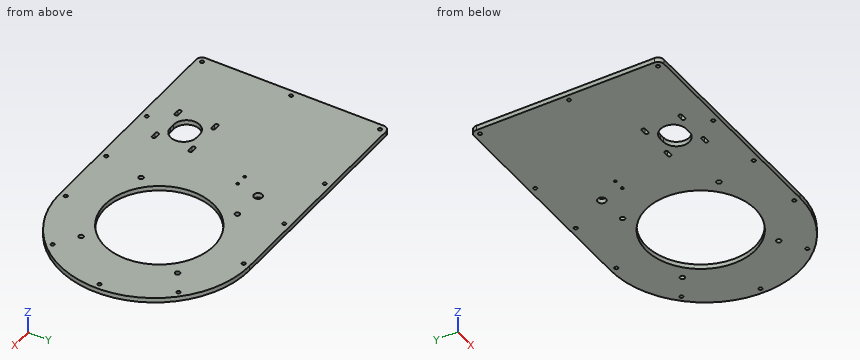
Autodesk Inventor part; units mm, degrees
ref_plane "YZ Plane" through (0, 0, 0) normal (1, 0, 0) x (0, 1, 0)
ref_plane "XZ Plane" through (0, 0, 0) normal (0, 1, 0) x (-1, 0, 0)
ref_plane "XY Plane" through (0, 0, 0) normal (0, 0, 1) x (1, 0, 0)
sketch "Sketch1" plane through (0, 0, 0) normal (0, 0, 1) x (1, 0, 0)
  line L0 (-150, -80) -> (40, -80)
  line L1 (40, 80) -> (-150, 80)
  line L2 (-150, 80) -> (-150, -80)
  line L3 (-150, 0) -> (-107, 0) construction
  line L4 (-107, 0) -> (33.79, 0) construction
  line L5 (33.79, -40.6) -> (33.79, 40.6) construction
  line L6 (-6.81, 0) -> (74.39, 0) construction
  line L7 (33.79, 40.6) -> (74.39, 40.6) construction
  line L8 (74.39, 40.6) -> (74.39, 0) construction
  circle A0 centre (74.39, 40.6) radius 2
  circle A1 centre (74.39, -40.6) radius 2
  circle A2 centre (-6.81, 40.6) radius 2
  circle A3 centre (-6.81, -40.6) radius 2
  line L9 (33.79, 0) -> (33.79, 47) construction
  line L10 (33.79, 0) -> (33.79, -47) construction
  line L11 (-107, -80) -> (-107, -42.5) construction
  line L12 (-107, -42.5) -> (-71.7142, -42.5) construction
  line L13 (33.79, 0) -> (-69.7142, -42.5) construction
  circle A4 centre (-69.7142, -42.5) radius 11 construction
  line L14 (150, 0) -> (120, 0) construction
  line L15 (120, 0) -> (120, 0)
  arc A5 (40, -80) -> (120, 0) centre (40, 0) ccw
  arc A6 (120, 0) -> (40, 80) centre (40, 0) ccw
  line L16 (120, 0) -> (115, 0) construction
  circle A7 centre (115, 0) radius 1.5
  line L17 (40, 0) -> (96.5685, 56.5685) construction
  line L18 (96.5685, -56.5685) -> (93.033, -53.033) construction
  circle A8 centre (93.033, -53.033) radius 1.5
  line L19 (40, -80) -> (40, -75) construction
  circle A9 centre (40, -75) radius 1.5
  line L20 (40, -75) -> (-15, -75) construction
  line L21 (-15, -75) -> (-70, -75) construction
  line L22 (-150, -75) -> (-145, -75) construction
  circle A10 centre (-15, -75) radius 1.5
  circle A11 centre (-70, -75) radius 1.5
  circle A12 centre (-145, -75) radius 1.5
  circle A13 centre (-145, 0) radius 1.5
  circle A14 centre (93.033, 53.033) radius 1.5
  circle A15 centre (40, 75) radius 1.5
  circle A16 centre (-15, 75) radius 1.5
  circle A17 centre (-70, 75) radius 1.5
  circle A18 centre (-145, 75) radius 1.5
  line L23 (-145, -80) -> (-145, -75) construction
  line L24 (-150, 0) -> (-145, 0) construction
  line L25 (-71.7142, -42.5) -> (-67.7142, -42.5) construction
  line L26 (-85.2142, -42.5) -> (-54.2142, -42.5) construction
  line L27 (-69.7142, -27) -> (-69.7142, -58) construction
  line L28 (-69.7142, -27) -> (-85.2142, -27) construction
  line L29 (-85.2142, -27) -> (-85.2142, -42.5) construction
  circle A19 centre (-85.2142, -27) radius 1.5 construction
  circle A20 centre (-54.2142, -27) radius 1.5 construction
  circle A21 centre (-54.2142, -58) radius 1.5 construction
  circle A22 centre (-85.2142, -58) radius 1.5 construction
  line L30 (33.79, 0) -> (31.29, 0) construction
  line L31 (33.79, 0) -> (45.79, 0) construction
  line L32 (45.79, 0) -> (45.79, 58) construction
  circle A23 centre (45.79, 58) radius 1.1
  circle A24 centre (45.79, 65) radius 1.1
  line L33 (-83.2142, -27) -> (-87.2142, -27) construction
  arc A25 (-83.2142, -28.5) -> (-83.2142, -25.5) centre (-83.2142, -27) ccw
  line L34 (-83.2142, -28.5) -> (-87.2142, -28.5)
  line L35 (-83.2142, -25.5) -> (-87.2142, -25.5)
  arc A26 (-87.2142, -25.5) -> (-87.2142, -28.5) centre (-87.2142, -27) ccw
  circle A27 centre (-54.2142, -27) radius 1.5 construction
  line L36 (-56.2142, -27) -> (-52.2142, -27) construction
  arc A28 (-56.2142, -25.5) -> (-56.2142, -28.5) centre (-56.2142, -27) ccw
  line L37 (-56.2142, -28.5) -> (-52.2142, -28.5)
  line L38 (-56.2142, -25.5) -> (-52.2142, -25.5)
  arc A29 (-52.2142, -28.5) -> (-52.2142, -25.5) centre (-52.2142, -27) ccw
  line L39 (-69.7142, -58) -> (-85.2142, -58) construction
  circle A30 centre (-85.2142, -58) radius 1.5 construction
  circle A31 centre (-54.2142, -58) radius 1.5 construction
  line L40 (-83.2142, -58) -> (-87.2142, -58) construction
  arc A32 (-83.2142, -59.5) -> (-83.2142, -56.5) centre (-83.2142, -58) ccw
  line L41 (-83.2142, -56.5) -> (-87.2142, -56.5)
  line L42 (-83.2142, -59.5) -> (-87.2142, -59.5)
  arc A33 (-87.2142, -56.5) -> (-87.2142, -59.5) centre (-87.2142, -58) ccw
  line L43 (-56.2142, -56.5) -> (-52.2142, -56.5)
  arc A34 (-52.2142, -59.5) -> (-52.2142, -56.5) centre (-52.2142, -58) ccw
  line L44 (-56.2142, -58) -> (-52.2142, -58) construction
  circle A35 centre (-54.2142, -58) radius 1.5 construction
  line L45 (-56.2142, -59.5) -> (-52.2142, -59.5)
  arc A36 (-56.2142, -56.5) -> (-56.2142, -59.5) centre (-56.2142, -58) ccw
  arc A37 (-71.7142, -31.5) -> (-71.7142, -53.5) centre (-71.7142, -42.5) ccw
  arc A38 (-67.7142, -53.5) -> (-67.7142, -31.5) centre (-67.7142, -42.5) ccw
  line L46 (-67.7142, -31.5) -> (-71.7142, -31.5)
  line L47 (-67.7142, -53.5) -> (-71.7142, -53.5)
  circle A39 centre (-37.21, 22) radius 1.1
  circle A40 centre (-46.71, 22) radius 1.1
  circle A41 centre (-32.71, 42) radius 3.5
  circle A42 centre (33.79, 0) radius 46
  point P0 (0, 0)
  point P1 (120, -80)
  point P2 (120, 0)
  dimension "d4" = 43
  dimension "d6" = 140.79
  dimension "L_furos" = 81.2
  dimension "d9" = 81.2
  dimension "d11" = 4
  dimension "d30" = 47
  dimension "d40" = 37.5
  dimension "d45" = 111.89
  dimension "DN" = 22
  dimension "d47" = 30
  dimension "d49" = 80
  dimension "LF" = 5
  dimension "Furos" = 3
  dimension "d52" = 45
  dimension "d53" = 5
  dimension "d55" = 3
  dimension "d56" = 5
  dimension "d57" = 3
  dimension "d58" = 55
  dimension "d59" = 55
  dimension "d60" = 5
  dimension "d61" = 3
  dimension "d62" = 3
  dimension "d63" = 3
  dimension "d64" = 3
  dimension "d65" = 5
  dimension "d66" = 5
  dimension "d67" = 33.79
  dimension "d68" = 4
  dimension "d69" = 31
  dimension "d70" = 31
  dimension "FN" = 3
  dimension "d72" = 2.5
  dimension "d77" = 12
  dimension "NN" = 4
  dimension "d84" = 3
  dimension "d85" = 1.5
  dimension "d86" = 22
  dimension "d88" = 11
  dimension "d89" = 43
  dimension "d90" = 58
  dimension "d91" = 7
  dimension "d92" = 2.2
  dimension "d93" = 2.2
  dimension "d94" = 80
  dimension "d95" = 80
  dimension "d96" = 40
  dimension "d97" = 150
  dimension "d98" = 2.2
  dimension "d99" = 2.2
  dimension "d100" = 9.5
  dimension "d101" = 22
  dimension "d102" = 71
  dimension "d103" = 20
  dimension "d104" = 7
  dimension "d106" = 14
  dimension "d107" = 92
extrude "Extrusion1" add sketch "Sketch1" along normal blind 4 contours L2 L1 A6 A5 L0 | A23 | A24 | A39 | A40 | A41
extrude "Extrusion5" cut sketch "Sketch1" along normal up to surface (4 mm away) contours A39 | A40 | A41
fillet "Fillet1" radius 5 2 edges at (-150, -80, 2) (-150, 80, 2)
equation "\"d9\" = L_furos"
equation "\"d53\" = LF"
equation "\"d55\" = Furos"
equation "\"d56\" = LF"
equation "\"d57\" = Furos"
equation "\"d60\" = LF"
equation "\"d61\" = Furos"
equation "\"d62\" = Furos"
equation "\"d63\" = Furos"
equation "\"d64\" = Furos"
equation "\"d65\" = LF"
equation "\"d66\" = LF"
properties part number "Base_solida_TestBR" material "Acrilico"
Model file for the job. Use its own axes, mm. Coordinates: 2 decimals unless noted, no trailing zeros. Loops run counter-clockwise (first coordinate to the right, second up) from the corner with the lowest first, then second, coordinate; pieces in that order, holes last. Notation, with made-up numbers: (0.5, 55.25) - (40.5, 55.25) arc R7 ccw to (40.5, 68.25) - close; hole circle Ø4 at (33.5, -28). An arc over 180 degrees is marked (long way). Answer as a JSON object with one key per item and string values. Group by question number.
(1) Cut at C-C (z = 3.2). State how many separate pieces and enclosed holes the cut face has, then the cut area to 3 significant figures.
(2) Cut at A-A (x = 33.79). Give the cut face in (y, z), then the cut area to 3 significant figures.
(3) Cut at B-B (y = 12). Give the cut face in (x, z).
(4) Cut at D-D (y = 61). Give the cut face in (x, z).
(5) Probe line 1 along Y through (x, z) = (-70, 1.8); line 2 along Y through (x, z) = (74.39, 2.85); line 3 along Y through (x, z) = (-37.21, 1.3). List the from-to ranges inside material, lowest first.
(6) Flat gauge pin, fed straight in: pin 1 (12 mm diameter, centred on x = 17, y = 32, fed in from -Z) (3 decimals). Where does the tip first touch, or does it go through?
Geometry says:
{
 "1": {"separate pieces": "1", "enclosed holes": "25", "area": "33,100 mm^2"},
 "2": {"outline": "(-80, 0) - (-46, 0) - (-46, 4) - (-80, 4) - close; (46, 0) - (80, 0) - (80, 4) - (46, 4) - close", "area": "272 mm^2"},
 "3": {"outline": "(-150, 0) - (-10.62, 0) - (-10.62, 4) - (-150, 4) - close; (78.2, 0) - (119.09, 0) - (119.09, 4) - (78.2, 4) - close"},
 "4": {"outline": "(-150, 0) - (91.76, 0) - (91.76, 4) - (-150, 4) - close"},
 "5": {"line 1": "y = -80 to -76.5, -73.5 to -53.5, -31.5 to 73.5, 76.5 to 80", "line 2": "y = -72.23 to -42.6, -38.6 to -21.62, 21.62 to 38.6, 42.6 to 72.23", "line 3": "y = -80 to 20.9, 23.1 to 80"},
 "6": {"pin 1": "passes through"}
}
